For this review, use the dimensioned drawing (mm, ordinates from the lowest corner) and the shaded views. A direction names the side the tool comes from. Round coordinates to 2 decimals unless told otherwise and drop trailing zeros. Write each loop counter-clockwise with the first axis right and the second up, starting at its lowest first coordinate (ties: lowest second). Pieces come first, ordered by that corner, then holes. Notation, with made-up numbers: (86, -37) -> (90, -37) arc R11 cw to (90, -33) -> close; hole circle Ø1 at (26.25, 60). An arc over 180 degrees is marked (long way). Write each question's results on one line, items separated by ' | '. Start each with the question number.
Item 1: Add section A-A (x = 98.1). State the section outline as (y, z) points, plus the area to 3 significant figures.
Item 2: Add section C-C (x = 60). State the section outline as (y, z) points.
Item 3: Tool access review of the marked faces 1 and 2: name each direction out of +Z, -Z, +X, -X, +Y, -Y from which nothing blocks a thin tool from reaching the whole face with its end or side.
Item 4: Add section B-B (z = 15). State the section outline as (x, y) points.
Item 5: Add section D-D (y = 24.25). State the section outline as (x, z) points, plus the area to 3 significant figures.
Item 6: To check wall thickness, follow line 1 along X through (y, z) = (1.9, 40); line 2 along Z through (x, y) = (98.1, 1.95); line 3 along Y through (x, z) = (69, 36). State the ranges of each line that lie inside material, in increasing order.
Item 7: Clearance check with flat-ended pins moving along their axes: pin 1 (4 mm diameter, centred on x = 53, z = 23.5, fed in from +Y); pin 2 (6 mm diameter, centred on x = 60.5, y = 9.5, fed in from -Z). State where each tip first meets the part, or that it passes through.
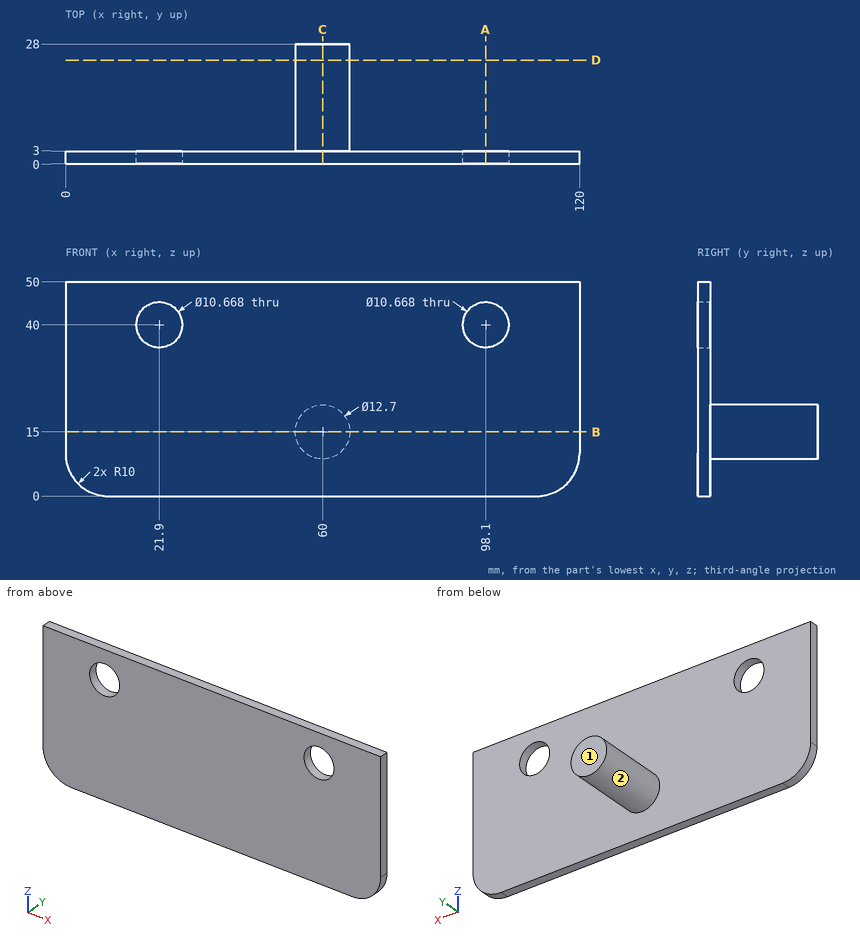
Responses:
1) outline: (0, 0) -> (3, 0) -> (3, 34.67) -> (0, 34.67) -> close; (0, 45.33) -> (3, 45.33) -> (3, 50) -> (0, 50) -> close | area: 118 mm^2
2) outline: (0, 0) -> (3, 0) -> (3, 8.65) -> (28, 8.65) -> (28, 21.35) -> (3, 21.35) -> (3, 50) -> (0, 50) -> close
3) face 1: +Z, -Z, +X, -X, +Y | face 2: +Y
4) outline: (0, 0) -> (120, 0) -> (120, 3) -> (66.35, 3) -> (66.35, 28) -> (53.65, 28) -> (53.65, 3) -> (0, 3) -> close
5) outline: circle Ø12.7 at (60, 15) | area: 127 mm^2
6) line 1: x = 0 to 16.57, 27.23 to 92.77, 103.43 to 120 | line 2: z = 0 to 34.67, 45.33 to 50 | line 3: y = 0 to 3
7) pin 1: stops at y = 3 | pin 2: stops at z = 8.65
